Verification items for the finished model (mm, model axes). Round coordinates to 2 decimals unless told otherwise and drop trailing zeros. Write each loop counter-clockwise with the first axis right and the second up, starting at its lowest first coordinate (ties: lowest second). Pieces come first, ordered by that corner, then holes.
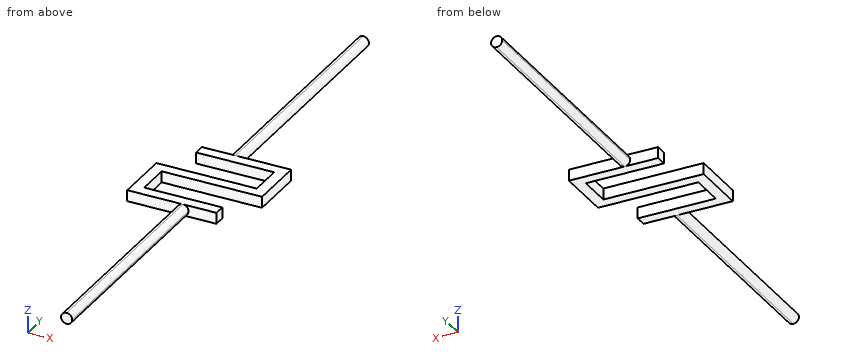
from build123d import *

# Parameters (mm, degrees)
F0_W      = 12.7
F0_H      = 12.7
F1_DEPTH  = 101.6
F2_W      = 38.1
F2_H      = 12.7
F2_W_2    = 12.7
F3_DEPTH  = 12.7
F4_W      = 38.1
F4_H      = 12.7
F4_W_2    = 12.7
F5_DEPTH  = 12.7
F6_W      = 88.9
F6_H      = 12.7
F6_W_2    = 12.7
F7_DEPTH  = 12.7
F8_W      = 88.9
F8_H      = 12.7
F8_W_2    = 12.7
F9_DEPTH  = 12.7
F11_DEPTH = 254
F13_DEPTH = 279.4


with BuildPart() as f1:
    # F0 (on Right) → F1 (new body)
    with BuildSketch(Plane.YZ):
        with Locations((-6.35, -6.35)):
            Rectangle(F0_W, F0_H)
    extrude(amount=F1_DEPTH)

    # F2 (on face) → F3 (join)
    with BuildSketch(Plane.YZ.offset(101.6)):
        with Locations((19.05, -6.35)):
            Rectangle(F2_W, F2_H)
        with Locations((-6.35, -6.35)):
            Rectangle(F2_W_2, F2_H)
    extrude(amount=F3_DEPTH)

    # F4 (on face) → F5 (join)
    with BuildSketch(Plane(origin=(0, 0, 0), x_dir=(0, -1, 0), z_dir=(-1, 0, 0))):
        with Locations((31.75, -6.35)):
            Rectangle(F4_W, F4_H)
        with Locations((6.35, -6.35)):
            Rectangle(F4_W_2, F4_H)
    extrude(amount=F5_DEPTH)

    # F6 (on face) → F7 (join)
    with BuildSketch(Plane.XZ.offset(50.8)):
        with Locations((44.45, -6.35)):
            Rectangle(F6_W, F6_H)
        with Locations((-6.35, -6.35)):
            Rectangle(F6_W_2, F6_H)
    extrude(amount=F7_DEPTH)

    # F8 (on face) → F9 (join)
    with BuildSketch(Plane(origin=(0, 38.1, 0), x_dir=(-1, 0, 0), z_dir=(0, 1, 0))):
        with Locations((-57.15, -6.35)):
            Rectangle(F8_W, F8_H)
        with Locations((-107.95, -6.35)):
            Rectangle(F8_W_2, F8_H)
    extrude(amount=F9_DEPTH)

    # F10 (on face) → F11 (join)
    with BuildSketch(Plane.XZ.offset(63.5)):
        with BuildLine():
            ThreePointArc((50.8, -12.7), (55.290128, -10.840128), (57.15, -6.35))
            ThreePointArc((57.15, -6.35), (55.290128, -1.859872), (50.8, 0))
            ThreePointArc((50.8, 0), (44.45, -6.35), (50.8, -12.7))
        make_face()
    extrude(amount=F11_DEPTH)

    # F12 (on face) → F13 (join)
    with BuildSketch(Plane(origin=(0, 50.8, 0), x_dir=(-1, 0, 0), z_dir=(0, 1, 0))):
        with BuildLine():
            ThreePointArc((-50.8, -12.7), (-46.309872, -10.840128), (-44.45, -6.35))
            ThreePointArc((-44.45, -6.35), (-46.309872, -1.859872), (-50.8, 0))
            ThreePointArc((-50.8, 0), (-57.15, -6.35), (-50.8, -12.7))
        make_face()
    extrude(amount=F13_DEPTH)


solid = f1.part
Q1. Sectioned sample at D-D (y = 122). Enter the section's corners in (x, z).
Recorded:
outline: circle Ø12.7 at (50.8, -6.35)
Q2. Depth check by flat-ended pin: P1, Ø3, axis at y = -117.5, z = -3.5, coming from the +X side; P2, Ø4, axis at y = 12.5, z = -4, coming from the -X side; P3, Ø4, axis at x = 41.5, z = -5, coming from the -Y side. Enter the tip coordinate at first touch or a pass-through.
Recorded:
P1: stops at x = 57
P2: stops at x = 101.6
P3: stops at y = -63.5
Q3. Sectioned sample at C-C (y = 32.5). Enter the section's corners in (x, z).
Recorded:
outline: (101.6, -12.7) - (114.3, -12.7) - (114.3, 0) - (101.6, 0) - close
Q4. Material ranges on line 1 along Y through (x, z) = (41, -5); line 2 along Y through (x, z) = (48.5, -4.75); line 3 along Y through (x, z) = (96, -3.5), recorded low to high.
Recorded:
line 1: y = -63.5 to -50.8, -12.7 to 0, 38.1 to 50.8
line 2: y = -317.5 to -50.8, -12.7 to 0, 38.1 to 330.2
line 3: y = -12.7 to 0, 38.1 to 50.8
Q5. Sectioned sample at B-B (z = -8.5). Enter the section's corners in (x, y).
Recorded:
outline: (-12.7, -63.5) - (44.83, -63.5) - (44.83, -317.5) - (56.77, -317.5) - (56.77, -63.5) - (88.9, -63.5) - (88.9, -50.8) - (0, -50.8) - (0, -12.7) - (114.3, -12.7) - (114.3, 50.8) - (56.77, 50.8) - (56.77, 330.2) - (44.83, 330.2) - (44.83, 50.8) - (12.7, 50.8) - (12.7, 38.1) - (101.6, 38.1) - (101.6, 0) - (-12.7, 0) - close
Q6. Sectioned sample at A-A (x = 29.5). Enter the section's corners in (y, z).
Recorded:
outline: (-63.5, -12.7) - (-50.8, -12.7) - (-50.8, 0) - (-63.5, 0) - close; (-12.7, -12.7) - (0, -12.7) - (0, 0) - (-12.7, 0) - close; (38.1, -12.7) - (50.8, -12.7) - (50.8, 0) - (38.1, 0) - close
